```python
from build123d import *

# Parameters (mm, degrees)
BOSS_EXTRUDE1_DEPTH = 7.5
SKETCH2_R           = 20
BOSS_EXTRUDE2_DEPTH = 20
CUT_EXTRUDE1_DEPTH  = 41


with BuildPart() as part:
    # Sketch1 → Boss-Extrude1 (new body, symmetric)
    with BuildSketch(Plane.XY):
        with BuildLine():
            Line((-1.5, 36), (1.5, 36))
            ThreePointArc((1.5, 36), (3.242504384, 33.062509074), (4, 29.732137495))
            ThreePointArc((4, 29.732137495), (5.85270966, 29.423558412), (7.682478298, 28.999647019))
            ThreePointArc((7.682478298, 28.999647019), (9.656791021, 31.786628134), (12.390784266, 33.833688319))
            Line((12.390784266, 33.833688319), (15.162422864, 32.685638022))
            ThreePointArc((15.162422864, 32.685638022), (15.64815789, 29.30492272), (15.073514558, 25.93817956))
            ThreePointArc((15.073514558, 25.93817956), (16.667106991, 24.944088369), (18.195368917, 23.852223166))
            ThreePointArc((18.195368917, 23.852223166), (21.085927531, 25.671521208), (24.395183951, 26.516504294))
            Line((24.395183951, 26.516504294), (26.516504294, 24.395183951))
            ThreePointArc((26.516504294, 24.395183951), (25.671521208, 21.085927531), (23.852223166, 18.195368917))
            ThreePointArc((23.852223166, 18.195368917), (24.944088369, 16.667106991), (25.93817956, 15.073514558))
            ThreePointArc((25.93817956, 15.073514558), (29.30492272, 15.64815789), (32.685638022, 15.162422864))
            Line((32.685638022, 15.162422864), (33.833688319, 12.390784266))
            ThreePointArc((33.833688319, 12.390784266), (31.786628134, 9.656791021), (28.999647019, 7.682478298))
            ThreePointArc((28.999647019, 7.682478298), (29.423558412, 5.85270966), (29.732137495, 4))
            ThreePointArc((29.732137495, 4), (33.062509074, 3.242504384), (36, 1.5))
            Line((36, 1.5), (36, -1.5))
            ThreePointArc((36, -1.5), (33.062509074, -3.242504384), (29.732137495, -4))
            ThreePointArc((29.732137495, -4), (29.423558412, -5.85270966), (28.999647019, -7.682478298))
            ThreePointArc((28.999647019, -7.682478298), (31.786628134, -9.656791021), (33.833688319, -12.390784266))
            Line((33.833688319, -12.390784266), (32.685638022, -15.162422864))
            ThreePointArc((32.685638022, -15.162422864), (29.30492272, -15.64815789), (25.93817956, -15.073514558))
            ThreePointArc((25.93817956, -15.073514558), (24.944088369, -16.667106991), (23.852223166, -18.195368917))
            ThreePointArc((23.852223166, -18.195368917), (25.671521208, -21.085927531), (26.516504294, -24.395183951))
            Line((26.516504294, -24.395183951), (24.395183951, -26.516504294))
            ThreePointArc((24.395183951, -26.516504294), (21.085927531, -25.671521208), (18.195368917, -23.852223166))
            ThreePointArc((18.195368917, -23.852223166), (16.667106991, -24.944088369), (15.073514558, -25.93817956))
            ThreePointArc((15.073514558, -25.93817956), (15.64815789, -29.30492272), (15.162422864, -32.685638022))
            Line((15.162422864, -32.685638022), (12.390784266, -33.833688319))
            ThreePointArc((12.390784266, -33.833688319), (9.656791021, -31.786628134), (7.682478298, -28.999647019))
            ThreePointArc((7.682478298, -28.999647019), (5.85270966, -29.423558412), (4, -29.732137495))
            ThreePointArc((4, -29.732137495), (3.242504384, -33.062509074), (1.5, -36))
            Line((1.5, -36), (-1.5, -36))
            ThreePointArc((-1.5, -36), (-3.242504384, -33.062509074), (-4, -29.732137495))
            ThreePointArc((-4, -29.732137495), (-5.85270966, -29.423558412), (-7.682478298, -28.999647019))
            ThreePointArc((-7.682478298, -28.999647019), (-9.656791021, -31.786628134), (-12.390784266, -33.833688319))
            Line((-12.390784266, -33.833688319), (-15.162422864, -32.685638022))
            ThreePointArc((-15.162422864, -32.685638022), (-15.64815789, -29.30492272), (-15.073514558, -25.93817956))
            ThreePointArc((-15.073514558, -25.93817956), (-16.667106991, -24.944088369), (-18.195368917, -23.852223166))
            ThreePointArc((-18.195368917, -23.852223166), (-21.085927531, -25.671521208), (-24.395183951, -26.516504294))
            Line((-24.395183951, -26.516504294), (-26.516504294, -24.395183951))
            ThreePointArc((-26.516504294, -24.395183951), (-25.671521208, -21.085927531), (-23.852223166, -18.195368917))
            ThreePointArc((-23.852223166, -18.195368917), (-24.944088369, -16.667106991), (-25.93817956, -15.073514558))
            ThreePointArc((-25.93817956, -15.073514558), (-29.30492272, -15.64815789), (-32.685638022, -15.162422864))
            Line((-32.685638022, -15.162422864), (-33.833688319, -12.390784266))
            ThreePointArc((-33.833688319, -12.390784266), (-31.786628134, -9.656791021), (-28.999647019, -7.682478298))
            ThreePointArc((-28.999647019, -7.682478298), (-29.423558412, -5.85270966), (-29.732137495, -4))
            ThreePointArc((-29.732137495, -4), (-33.062509074, -3.242504384), (-36, -1.5))
            Line((-36, -1.5), (-36, 1.5))
            ThreePointArc((-36, 1.5), (-33.062509074, 3.242504384), (-29.732137495, 4))
            ThreePointArc((-29.732137495, 4), (-29.423558412, 5.85270966), (-28.999647019, 7.682478298))
            ThreePointArc((-28.999647019, 7.682478298), (-31.786628134, 9.656791021), (-33.833688319, 12.390784266))
            Line((-33.833688319, 12.390784266), (-32.685638022, 15.162422864))
            ThreePointArc((-32.685638022, 15.162422864), (-29.30492272, 15.64815789), (-25.93817956, 15.073514558))
            ThreePointArc((-25.93817956, 15.073514558), (-24.944088369, 16.667106991), (-23.852223166, 18.195368917))
            ThreePointArc((-23.852223166, 18.195368917), (-25.671521208, 21.085927531), (-26.516504294, 24.395183951))
            Line((-26.516504294, 24.395183951), (-24.395183951, 26.516504294))
            ThreePointArc((-24.395183951, 26.516504294), (-21.085927531, 25.671521208), (-18.195368917, 23.852223166))
            ThreePointArc((-18.195368917, 23.852223166), (-16.667106991, 24.944088369), (-15.073514558, 25.93817956))
            ThreePointArc((-15.073514558, 25.93817956), (-15.64815789, 29.30492272), (-15.162422864, 32.685638022))
            Line((-15.162422864, 32.685638022), (-12.390784266, 33.833688319))
            ThreePointArc((-12.390784266, 33.833688319), (-9.656791021, 31.786628134), (-7.682478298, 28.999647019))
            ThreePointArc((-7.682478298, 28.999647019), (-5.85270966, 29.423558412), (-4, 29.732137495))
            ThreePointArc((-4, 29.732137495), (-3.242504384, 33.062509074), (-1.5, 36))
        make_face()
    extrude(amount=BOSS_EXTRUDE1_DEPTH, both=True)

    # Sketch2 → Boss-Extrude2 (add, symmetric)
    with BuildSketch(Plane.XY):
        Circle(SKETCH2_R)
    extrude(amount=BOSS_EXTRUDE2_DEPTH, both=True)

    # Sketch3 → Cut-Extrude1 (cut, through all)
    with BuildSketch(Plane.XY.offset(20)):
        with BuildLine():
            Line((-4, 15), (-4, 11.842719282))
            ThreePointArc((-4, 11.842719282), (0, -12.5), (4, 11.842719282))
            Line((4, 11.842719282), (4, 15))
            Line((4, 15), (-4, 15))
        make_face()
    extrude(amount=-CUT_EXTRUDE1_DEPTH, mode=Mode.SUBTRACT)


solid = part.part
```
Design review of the part built by this model. Coordinates are the model's own, in mm. A direction names the side the tool comes from. Coordinates: 2 decimals unless noted, no trailing zeros. Order: outer loops, then holes, each group sorted by start corner. A loop starts at its lowest first (then second) coordinate and runs counter-clockwise, first axis right, second up. Notation, with made-up numbers: M 3.5,18 L 7.5,18 A11 ccw 7.5,23 Z; hole C 38.25,50.25 d8. An arc over 180 degrees is marked long. Answer as a JSON object with one key per item and string values. Group by question number.
1) Add section B-B, the plane x = 0. Write out the cut boundary in (y, z).
2) Mouldability with a two-part tool opening along X and no side actions: class faces 1 (the cylindrical face through (5.88, -29.42, 0.11)), 2 (the cylindrical face through (-4.336, -19.524, -13.662)), 3 (the cylindrical face through (-29.257, -15.647, 0.105)), 4 (the cylindrical face through (-31.82, -9.69, 0.11)) as pulls with the +X half, pulls with the -X half, needs draft (parallel to the pull), parting line crosses it, or undercut.
3) Tool access review of faces 5 (the cylindrical face through (-9.69, 31.82, 0.11)), 6 (the cylindrical face through (-4.336, -19.524, 13.838)), 7 (the cylindrical face through (21.13, -25.69, 0.11)): name each direction out of +Z, -Z, +X, -X, +Y, -Y from which nothing blocks a thin tool from reaching the whole face with its end or side.
4) Add section A-A, the plane y = 0. Write out the cut boundary in (x, z), then the cut area to 3 significant figures.
5) Wall thickness on L1, parallel to X at y = 0, z = -3.5; L2, parallel to X at y = -32.5, z = 0.5; L3, parallel to Z at x = 26, y = -24: over which ranges is each line inside the solid? List them lowest first.
6) For pin 1 (1.5 mm diameter, centred on y = -10.5, z = -13.5, fed in from +X); pin 2 (1.6 mm diameter, centred on y = 14, z = -1.5, fed in from +X); pin 3 (1.5 mm diameter, centred on x = -2, y = 27, fed in from +Z), all flat-tipped, find the tip position at first contact; note any pin that passes through.
Computed values:
{
 "1": {"outline": "M -36,-7.5 L -20,-7.5 L -20,-20 L -12.5,-20 L -12.5,20 L -20,20 L -20,7.5 L -36,7.5 Z; M 15,-20 L 20,-20 L 20,-7.5 L 36,-7.5 L 36,7.5 L 20,7.5 L 20,20 L 15,20 Z"},
 "2": {"face 1": "undercut", "face 2": "parting line crosses it", "face 3": "undercut", "face 4": "pulls with the -X half"},
 "3": {"face 5": "+Z, -Z, +Y", "face 6": "+Z", "face 7": "+Z, -Z, -Y"},
 "4": {"outline": "M -36,-7.5 L -20,-7.5 L -20,-20 L -12.5,-20 L -12.5,20 L -20,20 L -20,7.5 L -36,7.5 Z; M 12.5,-20 L 20,-20 L 20,-7.5 L 36,-7.5 L 36,7.5 L 20,7.5 L 20,20 L 12.5,20 Z", "area": "1,080 mm^2"},
 "5": {"L1": "x = -36 to -12.5, 12.5 to 36", "L2": "x = -15.22 to -10.42, -3.45 to 3.45, 10.42 to 15.22", "L3": "z = -7.5 to 7.5"},
 "6": {"pin 1": "stops at x = 17.46", "pin 2": "stops at x = 33.5", "pin 3": "stops at z = 7.5"}
}
